Can you work these out from the model? Positions are in its coordinate system, mm. A direction names the side the tool comes from. Round coordinates to 2 decimals unless told otherwise and drop trailing zeros. Loops run counter-clockwise (first coordinate to the right, second up) from the corner with the lowest first, then second, coordinate; pieces in that order, holes last.
(1) I want a section at B-B on z = 4.45. Write out the boundary of the cut face in (x, y), plus the area to 3 significant figures.
(2) Which directions (+Z, -Z, +X, -X, +Y, -Y) give clear straight access to the entire face, cutting with the end or side of a thin tool? Please do faces 4 (the face through (5.5, -17, 4)), 5 (the face through (2, -5, 1)), 6 (the face through (56.27, -35.78, 3.83)).
(3) Thinking about a two-plate mould opening in X: for faces 1 (the face through (30, 0, 3)), 2 (the face through (39.94, -7.61, 0.54)), 3 (the face through (53.755, -31.94, 3.869)), which applies, released by +X, released by -X, zero draft, split by the parting line, or undercut?
(4) If I drill on line 1 along X through (y, z) = (-6.5, 2.75); line 2 along Z through (x, y) = (41.5, -4.5); line 3 along X through (y, z) = (-37, 4.5), over which ranges is the centre line in solid material (lowest first)?
(5) I want a section at A-A on y = -24.5. Write out the boundary of the cut face in (x, z).
(6) Will these pins go through, and if not, where does the flat tip stop? pin 1 Ø0.9 at (y, z) = (-4.5, 0.5) entering from +X; pin 2 Ø0.6 at (x, y) = (19, -20) entering from -Z; pin 3 Ø1.2 at (y, z) = (-4, 0.5) entering from -X.
from build123d import *

# Parameters (mm, degrees)
F1_DEPTH    = 2.5
F3_DEPTH    = 2.7
F4_R        = 1
F5_R        = 5
F7_R        = 2
F8_DEPTH    = 1
F6_W        = 8
F6_H        = 15
F9_DEPTH    = 1.1
F10_SIZE2   = 1.09999
F10_SIZE    = 14.99999
F10_2_SIZE2 = 1.09999
F10_2_SIZE  = 14.99999


# Not quite as in the source:
# - a fillet or chamfer that OpenCascade refuses, or shapes differently, is made with other operations: its cross-section is extruded or revolved along the edge and cut away or added
# - two fillets or chamfers of one size are made in one step
# - a fillet or chamfer is up to 0.001 mm smaller than in the source, because OpenCascade refuses the exact size


with BuildPart() as f1:
    # F0 (on Top) → F1 (new body)
    with BuildSketch(Plane.XY):
        Polygon((55, 0), (4, 0), (0, -10), (0, -47), (59, -47), (59, -10), align=None)
    extrude(amount=F1_DEPTH)

    # F2 (on face) → F3 (join)
    with BuildSketch(Plane.XY.offset(2.5)):
        with BuildLine():
            Line((0, -39.5), (0, -47))
            Line((0, -47), (59, -47))
            Line((59, -47), (59, -39.5))
            Line((59, -39.5), (53.5, -32))
            Line((53.5, -32), (53.5, -4))
            ThreePointArc((53.5, -4), (52.3284271247, -1.1715728753), (49.5, 0))
            Line((49.5, 0), (9.5, 0))
            ThreePointArc((9.5, 0), (6.6715728753, -1.1715728753), (5.5, -4))
            Line((5.5, -4), (5.5, -32))
            Line((5.5, -32), (0, -39.5))
        make_face()
    extrude(amount=F3_DEPTH)

    # F4
    f4_edges = [f1.edges().sort_by_distance(p)[0] for p in [
        (0, -47, 2.6),
        (59, -47, 2.6),
        (4, 0, 1.25),
        (55, 0, 1.25),
        (59, -10, 1.25),
        (0, -10, 1.25),
    ]]
    fillet(f4_edges, radius=F4_R)

    # F5
    f5_edges = [f1.edges().sort_by_distance(p)[0] for p in [
        (0, -39.5, 3.85),
        (59, -39.5, 3.85),
        (53.5, -32, 3.85),
        (5.5, -32, 3.85),
    ]]
    fillet(f5_edges, radius=F5_R)

    # F7 (on face) → F8 (cut)
    with BuildSketch(Plane(origin=(0, 0, 0), x_dir=(1, 0, 0), z_dir=(0, 0, -1))):
        with Locations((19, 20)):
            Circle(F7_R)
        with Locations((40, 20)):
            Circle(F7_R)
    extrude(amount=-F8_DEPTH, mode=Mode.SUBTRACT)

    # F6 (on face) → F9 (cut)
    with BuildSketch(Plane(origin=(0, 0, 0), x_dir=(1, 0, 0), z_dir=(0, 0, -1))):
        with Locations((40, 7.5)):
            Rectangle(F6_W, F6_H)
        with Locations((19, 7.5)):
            Rectangle(F6_W, F6_H)
    extrude(amount=-F9_DEPTH, mode=Mode.SUBTRACT)

    # F10 (size 15 and 1.1 in the source; OpenCascade refuses exactly that, so slightly less here)
    f10_edges = [f1.edges().sort_by_distance(p)[0] for p in [
        (40, -15, 1.1),
    ]]
    f10_side = f1.faces().sort_by_distance((40, -7.5, 1.1))[0]
    chamfer(f10_edges, length=F10_SIZE, length2=F10_SIZE2, reference=f10_side)

    # F10#2 (size 15 and 1.1 in the source; OpenCascade refuses exactly that, so slightly less here)
    f10_2_edges = [f1.edges().sort_by_distance(p)[0] for p in [
        (19, -15, 1.1),
    ]]
    f10_2_side = f1.faces().sort_by_distance((19, -7.5, 1.1))[0]
    chamfer(f10_2_edges, length=F10_2_SIZE, length2=F10_2_SIZE2, reference=f10_2_side)

    # F12: fillet of radius 2 on 2 edges, made by hand

    # F12_s1 → F12_t2 (revolve)
    with BuildSketch(Plane.XZ.offset(20)):
        with BuildLine():
            ThreePointArc((42, 0), (41.2679491924, 0.7320508076), (40.2679491924, 1))
            Line((40.2679491924, 1), (42, 1))
            Line((42, 1), (42, 0))
        make_face()
    revolve(axis=Axis((40, -20, 1), (0, 0, -1)))

    # F12_s3 → F12_t4 (revolve)
    with BuildSketch(Plane.XZ.offset(20)):
        with BuildLine():
            ThreePointArc((21, 0), (20.2679491924, 0.7320508076), (19.2679491924, 1))
            Line((19.2679491924, 1), (21, 1))
            Line((21, 1), (21, 0))
        make_face()
    revolve(axis=Axis((19, -20, 1), (0, 0, -1)))


solid = f1.part
Filled sheet:
1. outline: (0, -46) arc R1 ccw to (1, -47) - (58, -47) arc R1 ccw to (59, -46) - (59, -41.14) arc R5 ccw to (58.03, -38.18) - (54.47, -33.32) arc R5 cw to (53.5, -30.36) - (53.5, -4) arc R4 ccw to (49.5, 0) - (9.5, 0) arc R4 ccw to (5.5, -4) - (5.5, -30.36) arc R5 cw to (4.53, -33.32) - (0.97, -38.18) arc R5 ccw to (0, -41.14) - close
1. area: 2,370 mm2
2. face 4: +Z, -X, +Y
2. face 5: +Z, -Z, -X, +Y
2. face 6: +Z, +X, +Y
3. face 1: zero draft
3. face 2: undercut
3. face 3: released by +X
4. line 1: x = 5.5 to 53.5
4. line 2: z = 0.77 to 5.2
4. line 3: x = 1.83 to 57.17
5. outline: (0, 0) - (59, 0) - (59, 2.5) - (53.5, 2.5) - (53.5, 5.2) - (5.5, 5.2) - (5.5, 2.5) - (0, 2.5) - close
6. pin 1: stops at x = 56.98
6. pin 2: stops at z = 1
6. pin 3: stops at x = 2.16
